```python
from build123d import *

# Parameters (mm, degrees)
BOX028_W          = 15
BOX028_H          = 3
BOX028_DEPTH      = 3
BOX001_W          = 86
BOX001_H          = 2
BOX001_DEPTH      = 37
BOX002_W          = 86
BOX002_H          = 2
BOX002_DEPTH      = 37
BOX004_W          = 2
BOX004_H          = 70
BOX004_DEPTH      = 37
CYLINDER_R        = 1
CYLINDER_DEPTH    = 10
BOX005_W          = 13
BOX005_H          = 6.5
BOX005_DEPTH      = 37
CYLINDER001_R     = 1
CYLINDER001_DEPTH = 10
BOX007_W          = 13
BOX007_H          = 6.5
BOX007_DEPTH      = 37
CYLINDER002_R     = 1
CYLINDER002_DEPTH = 10
BOX006_W          = 15
BOX006_H          = 6.5
BOX006_DEPTH      = 37
BOX009_W          = 10
BOX009_H          = 10
BOX009_DEPTH      = 11
BOX010_W          = 16
BOX010_H          = 12
BOX010_DEPTH      = 11
BOX003_W          = 2
BOX003_H          = 70
BOX003_DEPTH      = 37
BOX018_W          = 15
BOX018_H          = 35
BOX018_DEPTH      = 10
BOX019_W          = 10
BOX019_H          = 20
BOX019_DEPTH      = 20
BOX020_W          = 10
BOX020_H          = 20
BOX020_DEPTH      = 20
BOX021_W          = 14
BOX021_H          = 20
BOX021_DEPTH      = 5
BOX022_W          = 14
BOX022_H          = 20
BOX022_DEPTH      = 5
BOX023_W          = 1.5
BOX023_H          = 5
BOX023_DEPTH      = 37
BOX024_W          = 1.5
BOX024_H          = 5
BOX024_DEPTH      = 37
BOX025_W          = 23
BOX025_H          = 10
BOX025_DEPTH      = 8
BOX016_W          = 86
BOX016_H          = 12
BOX016_DEPTH      = 10
BOX026_W          = 18
BOX026_H          = 10
BOX026_DEPTH      = 8
BOX017_W          = 86
BOX017_H          = 12
BOX017_DEPTH      = 10
BOX027_W          = 8
BOX027_H          = 5
BOX027_DEPTH      = 14
CYLINDER003_R     = 1
CYLINDER003_DEPTH = 10
BOX008_W          = 16
BOX008_H          = 6.5
BOX008_DEPTH      = 37
BOX_W             = 86
BOX_H             = 70
BOX_DEPTH         = 2
CHAMFER_SIZE      = 1


with BuildPart() as cubo028:
    # Box028 → Box028 (new body)
    with BuildSketch(Plane(origin=(35.5, 29, -1), x_dir=(1, 0, 0), z_dir=(0, 0, 1))):
        with Locations((7.5, 1.5)):
            Rectangle(BOX028_W, BOX028_H)
    extrude(amount=BOX028_DEPTH)


with BuildPart() as cubo001:
    # Box001 → Box001 (new body)
    with BuildSketch(Plane.XY):
        with Locations((43, 1)):
            Rectangle(BOX001_W, BOX001_H)
    extrude(amount=BOX001_DEPTH)


with BuildPart() as cubo002:
    # Box002 → Box002 (new body)
    with BuildSketch(Plane(origin=(0, 68, 0), x_dir=(1, 0, 0), z_dir=(0, 0, 1))):
        with Locations((43, 1)):
            Rectangle(BOX002_W, BOX002_H)
    extrude(amount=BOX002_DEPTH)


with BuildPart() as cubo004:
    # Box004 → Box004 (new body)
    with BuildSketch(Plane(origin=(84, 0, 0), x_dir=(1, 0, 0), z_dir=(0, 0, 1))):
        with Locations((1, 35)):
            Rectangle(BOX004_W, BOX004_H)
    extrude(amount=BOX004_DEPTH)


with BuildPart() as cilindro:
    # Cylinder → Cylinder (new body)
    with BuildSketch(Plane(origin=(3, 3, 27), x_dir=(1, 0, 0), z_dir=(0, 0, 1))):
        Circle(CYLINDER_R)
    extrude(amount=CYLINDER_DEPTH)


with BuildPart() as cut002:
    # Box005 → Box005 (new body)
    with BuildSketch(Plane.XY):
        with Locations((6.5, 3.25)):
            Rectangle(BOX005_W, BOX005_H)
    extrude(amount=BOX005_DEPTH)

    # Cut002: cut Cilindro
    add(cilindro.part, mode=Mode.SUBTRACT)


with BuildPart() as cilindro001:
    # Cylinder001 → Cylinder001 (new body)
    with BuildSketch(Plane(origin=(3, 67, 27), x_dir=(1, 0, 0), z_dir=(0, 0, 1))):
        Circle(CYLINDER001_R)
    extrude(amount=CYLINDER001_DEPTH)


with BuildPart() as cut003:
    # Box007 → Box007 (new body)
    with BuildSketch(Plane(origin=(0, 63.5, 0), x_dir=(1, 0, 0), z_dir=(0, 0, 1))):
        with Locations((6.5, 3.25)):
            Rectangle(BOX007_W, BOX007_H)
    extrude(amount=BOX007_DEPTH)

    # Cut003: cut Cilindro001
    add(cilindro001.part, mode=Mode.SUBTRACT)


with BuildPart() as cilindro002:
    # Cylinder002 → Cylinder002 (new body)
    with BuildSketch(Plane(origin=(83, 3, 27), x_dir=(1, 0, 0), z_dir=(0, 0, 1))):
        Circle(CYLINDER002_R)
    extrude(amount=CYLINDER002_DEPTH)


with BuildPart() as cut004:
    # Box006 → Box006 (new body)
    with BuildSketch(Plane(origin=(71, 0, 0), x_dir=(1, 0, 0), z_dir=(0, 0, 1))):
        with Locations((7.5, 3.25)):
            Rectangle(BOX006_W, BOX006_H)
    extrude(amount=BOX006_DEPTH)

    # Cut004: cut Cilindro002
    add(cilindro002.part, mode=Mode.SUBTRACT)


with BuildPart() as cubo009:
    # Box009 → Box009 (new body)
    with BuildSketch(Plane(origin=(-1, 9, 11.5), x_dir=(1, 0, 0), z_dir=(0, 0, 1))):
        with Locations((5, 5)):
            Rectangle(BOX009_W, BOX009_H)
    extrude(amount=BOX009_DEPTH)


with BuildPart() as cubo010:
    # Box010 → Box010 (new body)
    with BuildSketch(Plane(origin=(-1, 39, 11.5), x_dir=(1, 0, 0), z_dir=(0, 0, 1))):
        with Locations((8, 6)):
            Rectangle(BOX010_W, BOX010_H)
    extrude(amount=BOX010_DEPTH)


with BuildPart() as cut006:
    # Box003 → Box003 (new body)
    with BuildSketch(Plane.XY):
        with Locations((1, 35)):
            Rectangle(BOX003_W, BOX003_H)
    extrude(amount=BOX003_DEPTH)

    # Cut: cut Cubo010
    add(cubo010.part, mode=Mode.SUBTRACT)

    # Cut006: cut Cubo009
    add(cubo009.part, mode=Mode.SUBTRACT)


with BuildPart() as cubo018:
    # Box018 → Box018 (new body)
    with BuildSketch(Plane(origin=(70, 15, 0), x_dir=(1, 0, 0), z_dir=(0, 0, 1))):
        with Locations((7.5, 17.5)):
            Rectangle(BOX018_W, BOX018_H)
    extrude(amount=BOX018_DEPTH)


with BuildPart() as cubo019:
    # Box019 → Box019 (new body)
    with BuildSketch(Plane(origin=(25.5, 0, -20), x_dir=(1, 0, 0), z_dir=(0, 0, 1))):
        with Locations((5, 10)):
            Rectangle(BOX019_W, BOX019_H)
    extrude(amount=BOX019_DEPTH)


with BuildPart() as cubo020:
    # Box020 → Box020 (new body)
    with BuildSketch(Plane(origin=(50.5, 0, -20), x_dir=(1, 0, 0), z_dir=(0, 0, 1))):
        with Locations((5, 10)):
            Rectangle(BOX020_W, BOX020_H)
    extrude(amount=BOX020_DEPTH)


with BuildPart() as cubo021:
    # Box021 → Box021 (new body)
    with BuildSketch(Plane(origin=(25.5, 0, -20), x_dir=(1, 0, 0), z_dir=(0, 0, 1))):
        with Locations((7, 10)):
            Rectangle(BOX021_W, BOX021_H)
    extrude(amount=BOX021_DEPTH)


with BuildPart() as cubo022:
    # Box022 → Box022 (new body)
    with BuildSketch(Plane(origin=(46.5, 0, -20), x_dir=(1, 0, 0), z_dir=(0, 0, 1))):
        with Locations((7, 10)):
            Rectangle(BOX022_W, BOX022_H)
    extrude(amount=BOX022_DEPTH)


with BuildPart() as cubo023:
    # Box023 → Box023 (new body)
    with BuildSketch(Plane(origin=(82.5, 15, 0), x_dir=(1, 0, 0), z_dir=(0, 0, 1))):
        with Locations((0.75, 2.5)):
            Rectangle(BOX023_W, BOX023_H)
    extrude(amount=BOX023_DEPTH)


with BuildPart() as cubo024:
    # Box024 → Box024 (new body)
    with BuildSketch(Plane(origin=(82.5, 46, 0), x_dir=(1, 0, 0), z_dir=(0, 0, 1))):
        with Locations((0.75, 2.5)):
            Rectangle(BOX024_W, BOX024_H)
    extrude(amount=BOX024_DEPTH)


with BuildPart() as cubo025:
    # Box025 → Box025 (new body)
    with BuildSketch(Plane(origin=(41, 2, 2), x_dir=(1, 0, 0), z_dir=(0, 0, 1))):
        with Locations((11.5, 5)):
            Rectangle(BOX025_W, BOX025_H)
    extrude(amount=BOX025_DEPTH)


with BuildPart() as cut007:
    # Box016 → Box016 (new body)
    with BuildSketch(Plane.XY):
        with Locations((43, 6)):
            Rectangle(BOX016_W, BOX016_H)
    extrude(amount=BOX016_DEPTH)

    # Cut007: cut Cubo025
    add(cubo025.part, mode=Mode.SUBTRACT)


with BuildPart() as cubo026:
    # Box026 → Box026 (new body)
    with BuildSketch(Plane(origin=(58, 58, 2), x_dir=(1, 0, 0), z_dir=(0, 0, 1))):
        with Locations((9, 5)):
            Rectangle(BOX026_W, BOX026_H)
    extrude(amount=BOX026_DEPTH)


with BuildPart() as cut008:
    # Box017 → Box017 (new body)
    with BuildSketch(Plane(origin=(0, 58, 0), x_dir=(1, 0, 0), z_dir=(0, 0, 1))):
        with Locations((43, 6)):
            Rectangle(BOX017_W, BOX017_H)
    extrude(amount=BOX017_DEPTH)

    # Cut008: cut Cubo026
    add(cubo026.part, mode=Mode.SUBTRACT)


with BuildPart() as cubo027:
    # Box027 → Box027 (new body)
    with BuildSketch(Plane(origin=(70, 63, 2), x_dir=(1, 0, 0), z_dir=(0, 0, 1))):
        with Locations((4, 2.5)):
            Rectangle(BOX027_W, BOX027_H)
    extrude(amount=BOX027_DEPTH)


with BuildPart() as cilindro003:
    # Cylinder003 → Cylinder003 (new body)
    with BuildSketch(Plane(origin=(83, 67, 27), x_dir=(1, 0, 0), z_dir=(0, 0, 1))):
        Circle(CYLINDER003_R)
    extrude(amount=CYLINDER003_DEPTH)


with BuildPart() as cut009:
    # Box008 → Box008 (new body)
    with BuildSketch(Plane(origin=(70, 63.5, 0), x_dir=(1, 0, 0), z_dir=(0, 0, 1))):
        with Locations((8, 3.25)):
            Rectangle(BOX008_W, BOX008_H)
    extrude(amount=BOX008_DEPTH)

    # Cut005: cut Cilindro003
    add(cilindro003.part, mode=Mode.SUBTRACT)

    # Cut009: cut Cubo027
    add(cubo027.part, mode=Mode.SUBTRACT)


with BuildPart() as cut010:
    # Box → Box (new body)
    with BuildSketch(Plane.XY):
        with Locations((43, 35)):
            Rectangle(BOX_W, BOX_H)
    extrude(amount=BOX_DEPTH)

    # Fusion: union Cubo001, Cubo002, Cubo004, Cut002, Cut003, Cut004, Cut006, Cubo018, Cubo019, Cubo020, Cubo021, Cubo022, Cubo023, Cubo024, Cut007, Cut008, Cut009
    add(cubo001.part)
    add(cubo002.part)
    add(cubo004.part)
    add(cut002.part)
    add(cut003.part)
    add(cut004.part)
    add(cut006.part)
    add(cubo018.part)
    add(cubo019.part)
    add(cubo020.part)
    add(cubo021.part)
    add(cubo022.part)
    add(cubo023.part)
    add(cubo024.part)
    add(cut007.part)
    add(cut008.part)
    add(cut009.part)

    # Chamfer
    chamfer_edges = [cut010.edges().sort_by_distance(p)[0] for p in [
        (12.75, 0, 0),
        (43, 0, 0),
        (73.25, 0, 0),
        (86, 0, 18.5),
        (0, 0, 18.5),
        (0, 45, 11.5),
        (0, 51, 17),
        (0, 39, 17),
        (0, 45, 22.5),
        (0, 14, 11.5),
        (0, 19, 17),
        (0, 9, 17),
        (0, 14, 22.5),
        (0, 70, 18.5),
        (0, 35, 0),
        (43, 70, 0),
        (86, 35, 0),
        (77.5, 6.5, 10),
        (71, 4.25, 10),
        (67.5, 2, 10),
        (71, 2, 23.5),
        (25.5, 20, -10),
        (25.5, 10, -20),
        (60.5, 10, -20),
        (60.5, 20, -10),
        (32.5, 20, -20),
        (53.5, 20, -20),
        (86, 70, 18.5),
        (52.5, 2, 2),
        (77, 15, 2),
    ]]
    chamfer(chamfer_edges, length=CHAMFER_SIZE)

    # Cut010: cut Cubo028
    add(cubo028.part, mode=Mode.SUBTRACT)


solid = cut010.part
```
Part model, mm, in its own coordinate system. A direction names the side the tool comes from. Give positions to 0.01 mm unless a question says otherwise; leave off trailing zeros. Write each loop counter-clockwise with the first axis right and the second up, starting at its lowest first coordinate (ties: lowest second). Pieces come first, ordered by that corner, then holes. Notation, with made-up numbers: (-30.5, 24) -> (18.5, 24) arc R22 ccw to (18.5, 49) -> close; hole circle Ø2 at (67, 71). An arc over 180 degrees is marked (long way). Put each result on its own line as item: value. Start each with the question number.
Item 1: Cut at B-B (y = 44). List the corners of the cut face in (x, z), then the cut area to 3 significant figures.
Item 2: Pull direction Y, two halves, no side cores. Call faces 5 (the face through (35.5, 30, 1)), 6 (the face through (0, 35, 19)): pulls with the +Y half, pulls with the -Y half, needs draft (parallel to the pull), parting line crosses it, or undercut.
Item 3: Cut at C-C (x = 3). List the corners of the cut face in (y, z), then the cut area to 3 significant figures.
Item 4: Wall check: L1, parallel to X at y = 3, z = 32.75; L2, parallel to Y at x = 3, z = 30.75; L3, parallel to X at y = 67, z = 32. Give the ranges that are in metal, low to high. Write a range as [from, to].
Item 5: Pin check, flat tips, straight feed: pin 1 Ø2.5 at (y, z) = (47.5, 20) entering from -X; pin 2 Ø6 at (x, y) = (15, 34) entering from +Z; pin 3 Ø5.5 at (y, z) = (8, -17) entering from -X. Stop position of each tip, or through.
Item 6: Cut at A-A (z = -4). List the corners of the cut face in (x, y), then the cut area to 3 significant figures.
Item 7: Which spindle directions (+Z, -Z, +X, -X, +Y, -Y) get a long thin tool onto all of the face, cutting with end or side? Do faces 1 (the face through (33, 10, -20)), 2 (the face through (43, 29, 1)), 3 (the face through (30, 58, 6)), 4 (the face through (46.5, 10, -18)). Say none if no direction does.
Item 8: Cut at D-D (y = 67). List the corners of the cut face in (x, z), then the cut area to 3 significant figures.
Answer list:
1. outline: (0, 1) -> (1, 0) -> (85, 0) -> (86, 1) -> (86, 37) -> (84, 37) -> (84, 10) -> (70, 10) -> (70, 2) -> (2, 2) -> (2, 11.5) -> (1, 11.5) -> (0, 10.5) -> close; (0, 23.5) -> (1, 22.5) -> (2, 22.5) -> (2, 37) -> (0, 37) -> close
1. area: 400 mm2
2. face 5: undercut
2. face 6: needs draft
3. outline: (0, 1) -> (1, 0) -> (69, 0) -> (70, 1) -> (70, 37) -> (68, 37) -> (68, 27) -> (66, 27) -> (66, 37) -> (63.5, 37) -> (63.5, 10) -> (58, 10) -> (58, 2) -> (12, 2) -> (12, 10) -> (6.5, 10) -> (6.5, 37) -> (4, 37) -> (4, 27) -> (2, 27) -> (2, 37) -> (0, 37) -> close
3. area: 642 mm2
4. L1: x = [0, 2], [4, 13], [71, 82], [84, 86]
4. L2: y = [0, 2], [4, 6.5], [63.5, 66], [68, 70]
4. L3: x = [0, 2], [4, 13], [70, 82], [84, 86]
5. pin 1: stops at x = 82.5
5. pin 2: stops at z = 2
5. pin 3: stops at x = 25.5
6. outline: (25.5, 0) -> (35.5, 0) -> (35.5, 20) -> (26.5, 20) -> (25.5, 19) -> close; (50.5, 0) -> (60.5, 0) -> (60.5, 19) -> (59.5, 20) -> (50.5, 20) -> close
6. area: 399 mm2
7. face 1: -Z, +X, -X, +Y, -Y
7. face 2: +Z, -Z
7. face 3: +Z
7. face 4: -Z, +Y, -Y
8. outline: (0, 1) -> (1, 0) -> (85, 0) -> (86, 1) -> (86, 37) -> (84, 37) -> (84, 27) -> (82, 27) -> (82, 37) -> (70, 37) -> (70, 16) -> (78, 16) -> (78, 10) -> (76, 10) -> (76, 2) -> (58, 2) -> (58, 10) -> (13, 10) -> (13, 37) -> (4, 37) -> (4, 27) -> (2, 27) -> (2, 37) -> (0, 37) -> close
8. area: 1,410 mm2
